Geometry check sheet. Reference: the model listing, model coordinates, mm. Face numbers are marked on the shaded views. A direction names the side the tool comes from. Round coordinates to 2 decimals unless told otherwise and drop trailing zeros. Loops run counter-clockwise (first coordinate to the right, second up) from the corner with the lowest first, then second, coordinate; pieces in that order, holes last. Notation, with made-up numbers: (-1.5, -20.75) -> (54.5, -20.75) arc R11 cw to (54.5, -13.75) -> close; hole circle Ø10 at (-35, 82.5). An arc over 180 degrees is marked (long way). Use a Markdown table: item, result. Add a question column.
Q1. Gauge pin test, flat ends, axial feed: P1, Ø1, axis at x = -11, y = -7.5, coming from the -Z side; P2, Ø1.9, axis at x = 0, y = 5, coming from the -Z side; P3, Ø4.5, axis at x = 1, y = 14.5, coming from the -Z side. Record the tip position at first contact, or that the pin passes through.
Q2. Sectioned sample at B-B, the plane x = 0. Enter the section's corners in (y, z).
Q3. Sectioned sample at A-A, the plane z = 1. Enter the section's corners in (x, y).
Q4. Sectioned sample at D-D, the plane z = -14. Enter the section's corners in (x, y), then the cut area to 3 significant figures.
Q5. Material ranges on L1, parallel to Y at x = -10.5, z = -13; L2, parallel to Y at x = 0, z = 9; L3, parallel to Z at x = -19.05, y = -49.75, recorded low to high.
Q6. Sectioned sample at C-C, the plane y = 15. Enter the section's corners in (x, z).
Q7. Set-up check for the marked faces 1 and 2: record each of +Z, -Z, +X, -X, +Y, -Y from which the full face is reachable in a straight line by a thin tool's end or side.
Q8. Release check for a two-part mould opening along Y. For the marked faces 3, 4, 5 and 6 record: released by +Y, released by -Y, zero draft, split by the parting line, or undercut.
```python
from build123d import *

# Parameters (mm, degrees)
BOSS_EXTRUDE1_DEPTH         = 35.7124
F_10_CLEARANCE_HOLE1_D      = 4.9784
F_3_8_CLEARANCE_HOLE1_D     = 9.8044
F_3_8_CLEARANCE_HOLE1_DEPTH = 6.35


with BuildPart() as part:
    # Sketch1 → Boss-Extrude1 (new, symmetric)
    with BuildSketch(Plane(origin=(0, 0, 0), x_dir=(0, 0, -1), z_dir=(1, 0, 0))):
        Polygon((24.13, 27.178), (-12.7, 27.178), (-12.7, 0), (-12.7, -53.086), (25.4, -53.086), (25.4, -46.736), (0, -46.736), (0, 0), (24.13, 0), (24.13, 6.35), (-6.35, 6.35), (-6.35, 20.828), (24.13, 20.828), align=None)
    extrude(amount=BOSS_EXTRUDE1_DEPTH, both=True)

    # #10 Clearance Hole1 (through all)
    with Locations(Plane.XY.offset(12.7)):
        with Locations((0, 13.589)):
            Hole(F_10_CLEARANCE_HOLE1_D / 2)

    # 3/8 Clearance Hole1
    with Locations(Plane(origin=(0, -53.086, 0), x_dir=(-1, 0, 0), z_dir=(0, -1, 0))):
        with Locations((-19.05, 15.875), (19.05, 15.875)):
            Hole(F_3_8_CLEARANCE_HOLE1_D / 2, depth=F_3_8_CLEARANCE_HOLE1_DEPTH)


solid = part.part
```
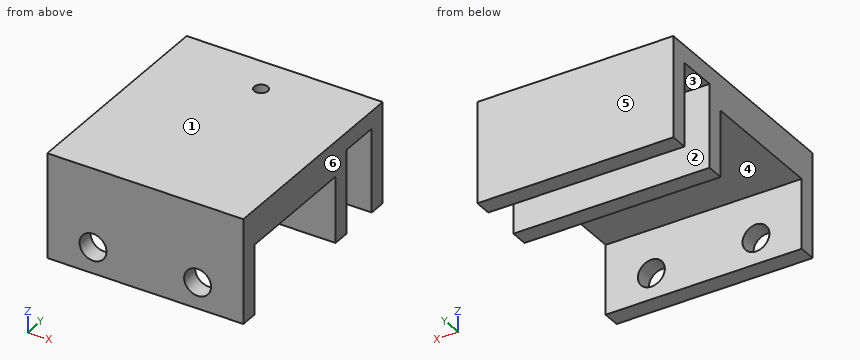
Values:
| question | item | result |
|---|---|---|
| 1 | P1 | z = 0 |
| 1 | P2 | z = -24.13 |
| 1 | P3 | z = 6.35 |
| 2 | outline | (-53.09, -25.4) -> (-46.74, -25.4) -> (-46.74, 0) -> (0, 0) -> (0, -24.13) -> (6.35, -24.13) -> (6.35, 6.35) -> (11.1, 6.35) -> (11.1, 12.7) -> (-53.09, 12.7) -> close; (16.08, 6.35) -> (20.83, 6.35) -> (20.83, -24.13) -> (27.18, -24.13) -> (27.18, 12.7) -> (16.08, 12.7) -> close |
| 3 | outline | (-35.71, -53.09) -> (35.71, -53.09) -> (35.71, 6.35) -> (-35.71, 6.35) -> close; (-35.71, 20.83) -> (35.71, 20.83) -> (35.71, 27.18) -> (-35.71, 27.18) -> close |
| 4 | outline | (-35.71, -53.09) -> (-23.58, -53.09) -> (-23.58, -46.74) -> (-35.71, -46.74) -> close; (-35.71, 0) -> (35.71, 0) -> (35.71, 6.35) -> (-35.71, 6.35) -> close; (-35.71, 20.83) -> (35.71, 20.83) -> (35.71, 27.18) -> (-35.71, 27.18) -> close; (-14.52, -53.09) -> (14.52, -53.09) -> (14.52, -46.74) -> (-14.52, -46.74) -> close; (23.58, -53.09) -> (35.71, -53.09) -> (35.71, -46.74) -> (23.58, -46.74) -> close |
| 4 | area | 1,250 mm^2 |
| 5 | L1 | -53.09 to -46.74, 0 to 6.35, 20.83 to 27.18 |
| 5 | L2 | -53.09 to 11.1, 16.08 to 27.18 |
| 5 | L3 | -25.4 to -20.78, -10.97 to 12.7 |
| 6 | outline | (-35.71, 6.35) -> (-2.05, 6.35) -> (-2.05, 12.7) -> (-35.71, 12.7) -> close; (2.05, 6.35) -> (35.71, 6.35) -> (35.71, 12.7) -> (2.05, 12.7) -> close |
| 7 | face 1 | +Z, +X, -X, +Y, -Y |
| 7 | face 2 | -Z, +X, -X |
| 8 | face 3 | undercut |
| 8 | face 4 | undercut |
| 8 | face 5 | released by +Y |
| 8 | face 6 | zero draft |
